The listing builds one solid part. Answer for the finished solid, in the listing's coordinates (mm). Face numbers are marked on the shaded views. A direction names the side the tool comes from. Give positions to 0.01 mm unless a question says otherwise; leave off trailing zeros. Loops run counter-clockwise (first coordinate to the right, second up) from the corner with the lowest first, then second, coordinate; pieces in that order, holes last. Notation, with made-up numbers: (76.5, -36) - (126.5, -36) arc R30 ccw to (126.5, -12) - close; hole circle Ø10 at (-27, 87.5). An arc over 180 degrees is marked (long way). Write item = value, one per line. Start each with the question number.
1) The part is cut by section A-A on x = 4.5. Write down the section's boundary in (y, z), plus the area to 3 significant figures.
2) The part is cut by section D-D on x = 31. Write down the section's boundary in (y, z).
3) The part is cut by section C-C on z = 1.45. Write down the section's boundary in (x, y).
4) Flat-ended cylindrical pins translate along their axes: P1, Ø2.5, axis at x = 18, z = 2.5, coming from the +Y side; P2, Ø1, axis at y = -5, z = 1, coming from the +X side; P3, Ø2, axis at y = -4.5, z = 4.5, coming from the -X side. Find the tip coordinate at first contact, or state that the pin passes through.
5) Consider probe 1 along X at (y, z) = (-0.25, 2.3); probe 2 along Y at (x, z) = (21.5, 1.15); probe 3 along Y at (x, z) = (9, 3.6). Determine where each line is inside the solid, lowest interval first.
6) The part is cut by section B-B on x = 27. Write down the section's boundary in (y, z).
7) The mould has two halves that part along Y. Classify the marked faces 1, 2 and 3: +Y half, -Y half, draft (parallel to the pull), parting line (faces both ways), or undercut.
8) Which of the six approach directions +Z, -Z, +X, -X, +Y, -Y give full straight-line access (tool end or side, diameter ignored) to the marked faces 4, 5 and 6?
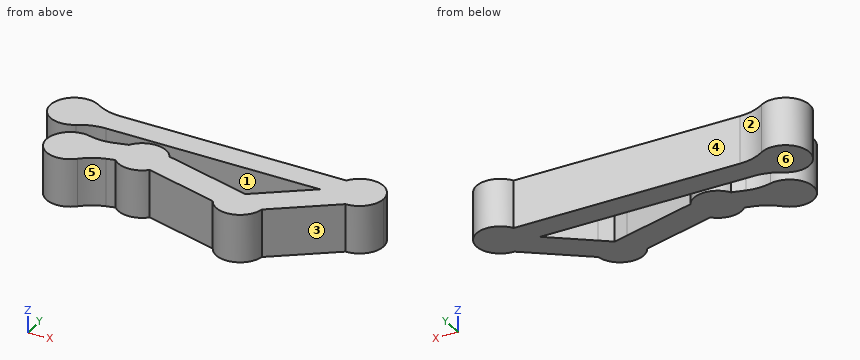
from build123d import *

# Parameters (mm, degrees)
F1_DEPTH = 5
F2_DEPTH = 5
F3_R     = 5


with BuildPart() as f1:
    # F0 (on Top) → F1 (new body)
    with BuildSketch(Plane.XY):
        with BuildLine():
            ThreePointArc((3.8778323824, 0.876766336), (4.1491402261, 0.2522371821), (4.2418691481, -0.4223337609))
            ThreePointArc((4.2418691481, -0.4223337609), (4.1491402261, -1.0969047038), (3.8778323824, -1.7214338577))
            Line((3.8778323824, -1.7214338577), (28.311316439, -1.7214338577))
            Line((28.311316439, -1.7214338577), (29.302722756, -0.9705717363))
            ThreePointArc((29.302722756, -0.9705717363), (29.2748726925, -0.0174529288), (29.6059059138, 0.876766336))
            Line((29.6059059138, 0.876766336), (3.8778323824, 0.876766336))
        make_face()
        with BuildLine():
            ThreePointArc((34.2418691481, -0.4223337609), (32.4164400911, 1.9849373171), (29.6059059138, 0.876766336))
            Line((29.6059059138, 0.876766336), (31.7418691481, 0.876766336))
            Line((31.7418691481, 0.876766336), (33.5531306582, -1.5147461023))
            Line((33.5531306582, -1.5147461023), (31.6951874639, -2.921897887))
            ThreePointArc((31.6951874639, -2.921897887), (33.4930538599, -2.206528847), (34.2418691481, -0.4223337609))
        make_face()
        with BuildLine():
            Line((33.5531306582, -1.5147461023), (31.7418691481, 0.876766336))
            Line((31.7418691481, 0.876766336), (31.7418691481, -1.7214338577))
            Line((31.7418691481, -1.7214338577), (29.6059059138, -1.7214338577))
            ThreePointArc((29.6059059138, -1.7214338577), (30.4963719858, -2.5899907491), (31.6951874639, -2.921897887))
            Line((31.6951874639, -2.921897887), (33.5531306582, -1.5147461023))
        make_face()
        with BuildLine():
            Line((31.7418691481, 0.876766336), (29.6059059138, 0.876766336))
            ThreePointArc((29.6059059138, 0.876766336), (29.2748726925, -0.0174529288), (29.302722756, -0.9705717363))
            Line((29.302722756, -0.9705717363), (31.7418691481, 0.876766336))
        make_face()
        with BuildLine():
            Line((31.7418691481, -1.7214338577), (31.7418691481, 0.876766336))
            Line((31.7418691481, 0.876766336), (29.302722756, -0.9705717363))
            ThreePointArc((29.302722756, -0.9705717363), (29.4237113655, -1.358359666), (29.6059059138, -1.7214338577))
            Line((29.6059059138, -1.7214338577), (31.7418691481, -1.7214338577))
        make_face()
        with BuildLine():
            Line((29.6059059138, -1.7214338577), (28.311316439, -1.7214338577))
            Line((28.311316439, -1.7214338577), (24.0527407032, -4.9467544517))
            ThreePointArc((24.0527407032, -4.9467544517), (25.1599747934, -5.8682005046), (25.5749808252, -7.2476207279))
            ThreePointArc((25.5749808252, -7.2476207279), (25.569649156, -7.4108074897), (25.5536768898, -7.5732982052))
            Line((25.5536768898, -7.5732982052), (31.6951874639, -2.921897887))
            ThreePointArc((31.6951874639, -2.921897887), (30.4963719858, -2.5899907491), (29.6059059138, -1.7214338577))
        make_face()
        with BuildLine():
            Line((29.302722756, -0.9705717363), (28.311316439, -1.7214338577))
            Line((28.311316439, -1.7214338577), (29.6059059138, -1.7214338577))
            ThreePointArc((29.6059059138, -1.7214338577), (29.4237113655, -1.358359666), (29.302722756, -0.9705717363))
        make_face()
        with BuildLine():
            ThreePointArc((25.5749808252, -7.2476207279), (25.1599747934, -5.8682005046), (24.0527407032, -4.9467544517))
            Line((24.0527407032, -4.9467544517), (22.8393681886, -5.8657272732))
            Line((22.8393681886, -5.8657272732), (24.2570694169, -6.2455991724))
            Line((24.2570694169, -6.2455991724), (23.4806122816, -9.1433766513))
            Line((23.4806122816, -9.1433766513), (25.5536768898, -7.5732982052))
            ThreePointArc((25.5536768898, -7.5732982052), (25.569649156, -7.4108074897), (25.5749808252, -7.2476207279))
        make_face()
        with BuildLine():
            ThreePointArc((20.8814307518, -8.4469280594), (23.5344743938, -9.7050310844), (25.5536768898, -7.5732982052))
            Line((25.5536768898, -7.5732982052), (23.4806122816, -9.1433766513))
            Line((23.4806122816, -9.1433766513), (20.8814307518, -8.4469280594))
        make_face()
        with BuildLine():
            Line((21.6693507715, -6.751864213), (22.8393681886, -5.8657272732))
            Line((22.8393681886, -5.8657272732), (21.3268372671, -5.4604458343))
            ThreePointArc((21.3268372671, -5.4604458343), (20.6023291733, -6.8788473441), (20.8814307518, -8.4469280594))
            Line((20.8814307518, -8.4469280594), (23.4806122816, -9.1433766513))
            Line((23.4806122816, -9.1433766513), (21.6693507715, -6.751864213))
        make_face()
        Polygon((24.2570694169, -6.2455991724), (22.8393681886, -5.8657272732), (21.6693507715, -6.751864213), (23.4806122816, -9.1433766513), align=None)
        with BuildLine():
            ThreePointArc((20.8814307518, -8.4469280594), (20.6023291733, -6.8788473441), (21.3268372671, -5.4604458343))
            Line((21.3268372671, -5.4604458343), (13.4219767307, -3.3423448372))
            ThreePointArc((13.4219767307, -3.3423448372), (13.6767457968, -3.9504448184), (13.7636843696, -4.6040001325))
            ThreePointArc((13.7636843696, -4.6040001325), (13.5793417545, -5.5461948448), (13.0534996689, -6.3494402473))
            Line((13.0534996689, -6.3494402473), (20.8814307518, -8.4469280594))
        make_face()
        with BuildLine():
            ThreePointArc((13.7636843696, -4.6040001325), (13.6767457968, -3.9504448184), (13.4219767307, -3.3423448372))
            Line((13.4219767307, -3.3423448372), (11.4246112089, -2.8071523587))
            Line((11.4246112089, -2.8071523587), (12.1704041891, -5.5904896527))
            Line((12.1704041891, -5.5904896527), (11.1957308392, -5.8516525897))
            Line((11.1957308392, -5.8516525897), (13.0534996689, -6.3494402473))
            ThreePointArc((13.0534996689, -6.3494402473), (13.5793417545, -5.5461948448), (13.7636843696, -4.6040001325))
        make_face()
        with BuildLine():
            Line((11.4246112089, -2.8071523587), (13.4219767307, -3.3423448372))
            ThreePointArc((13.4219767307, -3.3423448372), (11.2889517228, -2.1041278236), (9.1313345982, -3.2989773541))
            Line((9.1313345982, -3.2989773541), (11.3939470538, -2.6927121739))
            Line((11.3939470538, -2.6927121739), (11.4246112089, -2.8071523587))
        make_face()
        with BuildLine():
            Line((11.2012257233, -2.7472963982), (11.4246112089, -2.8071523587))
            Line((11.4246112089, -2.8071523587), (11.3939470538, -2.6927121739))
            Line((11.3939470538, -2.6927121739), (9.1313345982, -3.2989773541))
            ThreePointArc((9.1313345982, -3.2989773541), (8.7771380409, -4.8630124006), (9.44607009, -6.3204727745))
            Line((9.44607009, -6.3204727745), (11.1957308392, -5.8516525897))
            Line((11.1957308392, -5.8516525897), (10.424768588, -5.6450738771))
            Line((10.424768588, -5.6450738771), (11.2012257233, -2.7472963982))
        make_face()
        Polygon((12.1704041891, -5.5904896527), (11.4246112089, -2.8071523587), (11.2012257233, -2.7472963982), (10.424768588, -5.6450738771), (11.1957308392, -5.8516525897), align=None)
        with BuildLine():
            ThreePointArc((9.44607009, -6.3204727745), (11.2436101462, -7.1039195363), (13.0534996689, -6.3494402473))
            Line((13.0534996689, -6.3494402473), (11.1957308392, -5.8516525897))
            Line((11.1957308392, -5.8516525897), (9.44607009, -6.3204727745))
        make_face()
        with BuildLine():
            ThreePointArc((9.44607009, -6.3204727745), (8.7771380409, -4.8630124006), (9.1313345982, -3.2989773541))
            Line((9.1313345982, -3.2989773541), (6.1034072345, -4.110308046))
            ThreePointArc((6.1034072345, -4.110308046), (6.8080120864, -4.9834588452), (7.0597841495, -6.0768348756))
            ThreePointArc((7.0597841495, -6.0768348756), (7.0143921173, -6.5510708134), (6.8798643698, -7.0080855248))
            Line((6.8798643698, -7.0080855248), (9.44607009, -6.3204727745))
        make_face()
        with BuildLine():
            Line((4.1715555819, -4.6279461362), (6.1034072345, -4.110308046))
            ThreePointArc((6.1034072345, -4.110308046), (2.1449695838, -6.7238824884), (6.8798643698, -7.0080855248))
            Line((6.8798643698, -7.0080855248), (4.9480127172, -7.525723615))
            Line((4.9480127172, -7.525723615), (4.1715555819, -4.6279461362))
        make_face()
        with BuildLine():
            ThreePointArc((7.0597841495, -6.0768348756), (6.8080120864, -4.9834588452), (6.1034072345, -4.110308046))
            Line((6.1034072345, -4.110308046), (4.1715555819, -4.6279461362))
            Line((4.1715555819, -4.6279461362), (4.9480127172, -7.525723615))
            Line((4.9480127172, -7.525723615), (6.8798643698, -7.0080855248))
            ThreePointArc((6.8798643698, -7.0080855248), (7.0143921173, -6.5510708134), (7.0597841495, -6.0768348756))
        make_face()
    extrude(amount=F1_DEPTH)

    # F0 (on Top) → F2 (join)
    with BuildSketch(Plane.XY):
        with BuildLine():
            Line((1.7418691481, 0.876766336), (3.8778323824, 0.876766336))
            ThreePointArc((3.8778323824, 0.876766336), (-0.7581308519, -0.4223337609), (3.8778323824, -1.7214338577))
            Line((3.8778323824, -1.7214338577), (1.7418691481, -1.7214338577))
            Line((1.7418691481, -1.7214338577), (1.7418691481, 0.876766336))
        make_face()
        with BuildLine():
            ThreePointArc((3.8778323824, -1.7214338577), (4.1491402261, -1.0969047038), (4.2418691481, -0.4223337609))
            ThreePointArc((4.2418691481, -0.4223337609), (4.1491402261, 0.2522371821), (3.8778323824, 0.876766336))
            Line((3.8778323824, 0.876766336), (1.7418691481, 0.876766336))
            Line((1.7418691481, 0.876766336), (1.7418691481, -1.7214338577))
            Line((1.7418691481, -1.7214338577), (3.8778323824, -1.7214338577))
        make_face()
    extrude(amount=F2_DEPTH)

    # F3
    f3_edges = [f1.edges().sort_by_distance(p)[0] for p in [
        (3.877832, 0.876766, 2.5),
        (3.877832, -1.721434, 2.5),
        (6.879864, -7.008086, 2.5),
        (6.103407, -4.110308, 2.5),
    ]]
    fillet(f3_edges, radius=F3_R)


solid = f1.part
Answer below:
q1.outline = (-8.58, 0) - (-3.58, 0) - (-3.58, 5) - (-8.58, 5) - close; (-1.9, 0) - (1.05, 0) - (1.05, 5) - (-1.9, 5) - close
q1.area = 39.7 mm2
q2.outline = (-3.45, 0) - (1.97, 0) - (1.97, 5) - (-3.45, 5) - close
q3.outline = (3.1, -2.52) arc R5 cw to (5.81, -1.72) - (28.31, -1.72) - (22.84, -5.87) - (13.42, -3.34) arc R2.5 ccw to (9.13, -3.3) - (7.79, -3.66) arc R5 cw to (5.2, -3.66) arc R2.5 ccw (long way) to (6.33, -7.85) arc R5 cw to (8.56, -6.56) - (9.45, -6.32) arc R2.5 ccw to (13.05, -6.35) - (20.88, -8.45) arc R2.5 ccw to (25.55, -7.57) - (31.7, -2.92) arc R2.5 ccw (long way) to (29.61, 0.88) - (5.81, 0.88) arc R5 cw to (3.1, 1.68) arc R2.5 ccw (long way) to start
q4.P1 = 0.88
q4.P2 = 29.61
q4.P3 = 2.13
q5.probe_1 = -0.75 to 34.24
q5.probe_2 = -9.19 to -5.51, -1.72 to 0.88
q5.probe_3 = -6.44 to -3.33, -1.72 to 0.88
q6.outline = (-6.48, 0) - (-2.71, 0) - (-2.71, 5) - (-6.48, 5) - close; (-1.72, 0) - (0.88, 0) - (0.88, 5) - (-1.72, 5) - close
q7.face_1 = undercut
q7.face_2 = +Y half
q7.face_3 = -Y half
q8.face_4 = +Z, -Z, +Y
q8.face_5 = +Z, -Z, -Y
q8.face_6 = -Z, +X, -X, +Y, -Y
